The listing builds one solid part. Answer for the finished solid, in the listing's coordinates (mm). A direction names the side the tool comes from. Coordinates: 2 decimals unless noted, no trailing zeros. Order: outer loops, then holes, each group sorted by start corner. A loop starts at its lowest first (then second) coordinate and runs counter-clockwise, first axis right, second up. Notation, with made-up numbers: (3.25, -14.5) -> (17.25, -14.5) arc R32 ccw to (17.25, 13.5) -> close; hole circle Ø7 at (64.5, -28). An arc over 180 degrees is marked (long way). One line per question, with ' | ' between items.
from build123d import *

# Parameters (mm, degrees)
SKETCH1_R                        = 65.405
SKETCH1_R_2                      = 63.5
BOSS_EXTRUDE1_DEPTH              = 25.4
F_5_8_0_625_DIAMETER_HOLE1_D     = 15.875
F_5_8_0_625_DIAMETER_HOLE1_DEPTH = 3.81
F_5_8_0_625_DIAMETER_HOLE2_D     = 15.875
F_5_8_0_625_DIAMETER_HOLE2_DEPTH = 3.81


with BuildPart() as part:
    # Sketch1 → Boss-Extrude1 (new body, symmetric)
    with BuildSketch(Plane(origin=(0, 0, 0), x_dir=(1, 0, 0), z_dir=(0, 1, 0))):
        Circle(SKETCH1_R)
        Circle(SKETCH1_R_2, mode=Mode.SUBTRACT)
    extrude(amount=BOSS_EXTRUDE1_DEPTH, both=True)

    # 5/8 (0.625) Diameter Hole1
    with Locations(Plane(origin=(56.642391535, 0, -32.7025), x_dir=(0, -1, 0), z_dir=(0.866025404, 0, -0.5))):
        with Locations((0, 0)):
            Hole(F_5_8_0_625_DIAMETER_HOLE1_D / 2, depth=F_5_8_0_625_DIAMETER_HOLE1_DEPTH)

    # 5/8 (0.625) Diameter Hole2
    with Locations(Plane.XY.offset(65.405)):
        with Locations((0, 0)):
            Hole(F_5_8_0_625_DIAMETER_HOLE2_D / 2, depth=F_5_8_0_625_DIAMETER_HOLE2_DEPTH)


solid = part.part
Item 1: For faces 4 (the face through (-7.571, 2.384, 64.187)), 5 (the face through (-54, 25.4, -34)), determine the directions among +Z, -Z, +X, -X, +Y, -Y from which every point of the face is accessible in a straight line to the end or side of a thin tool.
Computed values:
face 4: +Z | face 5: +Z, -Z, +X, -X, +Y
Item 2: Section D-D, the plane y = -17.5 is taken. Give the vertices of the cut face in (x, z) (3 decimals).
Computed values:
outline: circle Ø130.81 at (0, 0); hole circle Ø127 at (0, 0)
Item 3: Section C-C, the plane y = 6 is taken. Give the vertices of the cut face in (x, z) (3 decimals).
Computed values:
outline: (-5.197, 63.287) -> (-5.197, 65.198) arc R65.405 ccw (long way) to (53.865, -37.099) -> (52.21, -36.144) arc R63.5 cw (long way) to start; (5.197, 63.287) arc R63.5 cw to (57.406, -27.143) -> (59.062, -28.099) arc R65.405 ccw to (5.197, 65.198) -> close
Item 4: Section A-A, the plane x = 0 is taken. Give the vertices of the cut face in (y, z) (1 decimal), plus the area to 3 significant figures.
Computed values:
outline: (-25.4, -65.4) -> (25.4, -65.4) -> (25.4, -63.5) -> (-25.4, -63.5) -> close; (-25.4, 63.5) -> (-7.9, 63.5) -> (-7.9, 65.4) -> (-25.4, 65.4) -> close; (7.9, 63.5) -> (25.4, 63.5) -> (25.4, 65.4) -> (7.9, 65.4) -> close | area: 163 mm^2
Item 5: Find the intervals of material crossed by L1, parallel to Y at x = 0, z = 64.75; L2, parallel to X at y = 5, z = -52.5; L3, parallel to Z at x = -49.5, y = 8.5, in increasing order.
Computed values:
L1: y = -25.4 to -7.94, 7.94 to 25.4 | L2: x = -39.01 to -35.72, 35.72 to 39.01 | L3: z = -42.75 to -39.77, 39.77 to 42.75
Item 6: Each of these flat-tipped pins is pushed along its axis until it touches: pin 1 Ø10 at (x, y) = (49.5, -5.5) entering from +Z; pin 2 Ø3 at (x, y) = (2.5, 13) entering from +Z; pin 3 Ø4 at (y, z) = (20, 33.5) entering from +X. Where does it stop, or does it pass through?
Computed values:
pin 1: stops at z = 47.93 | pin 2: stops at z = 65.4 | pin 3: stops at x = 57.32
Item 7: Determine the mould class of faces 1 (the face through (59.108, 3.663, -25.995)), 2 (the face through (-54, -25.4, -34)), 3 (the face through (-14.18, 0.36, 63.85)) for opening direction X: pulls with the +X half, pulls with the -X half, needs draft (parallel to the pull), parting line crosses it, or undercut.
Computed values:
face 1: undercut | face 2: needs draft | face 3: parting line crosses it
Item 8: Section B-B, the plane z = 0 is taken. Give the vertices of the cut face in (x, y) (3 decimals), plus the area to 3 significant figures.
Computed values:
outline: (-65.405, -25.4) -> (-63.5, -25.4) -> (-63.5, 25.4) -> (-65.405, 25.4) -> close; (63.5, -25.4) -> (65.405, -25.4) -> (65.405, 25.4) -> (63.5, 25.4) -> close | area: 194 mm^2
